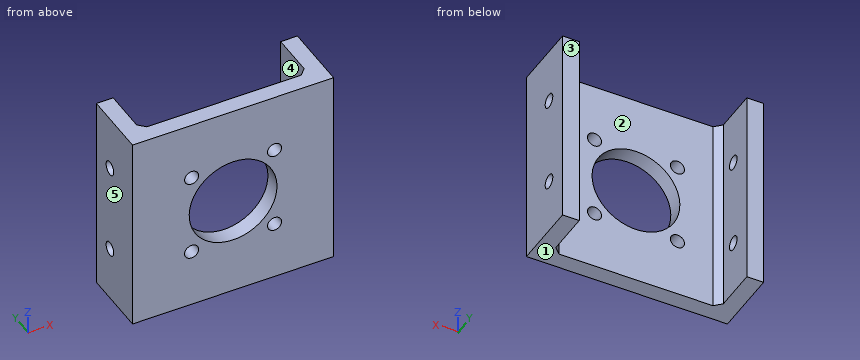
```python
from build123d import *

# Parameters (mm, degrees)
SKETCH_1_W           = 60
SKETCH_1_H           = 60
SKETCH_1_R           = 13.1
SKETCH_1_R_2         = 2.1
EXTRUDE_1_DEPTH      = 5
SKETCH_2_W           = 5
SKETCH_2_H           = 60
EXTRUDE_2_DEPTH      = 15
SKETCH_4_R           = 2.1
CUT_EXTRUDE_M4_DEPTH = 71
CHAMFER_1_SIZE       = 2


with BuildPart() as part:
    # 草图1 → 凸台-拉伸1 (new body)
    with BuildSketch(Plane(origin=(0, 0, 0), x_dir=(1, 0, 0), z_dir=(0, 1, 0))):
        Rectangle(SKETCH_1_W, SKETCH_1_H)
        with Locations(Location((0, 0, 0), (0, 0, 270))):
            Circle(SKETCH_1_R, mode=Mode.SUBTRACT)
        with Locations(Location((-12.374368671, -12.374368671, 0), (0, 0, 270))):
            Circle(SKETCH_1_R_2, mode=Mode.SUBTRACT)
        with Locations(Location((12.374368671, -12.374368671, 0), (0, 0, 90))):
            Circle(SKETCH_1_R_2, mode=Mode.SUBTRACT)
        with Locations(Location((-12.374368671, 12.374368671, 0), (0, 0, 90))):
            Circle(SKETCH_1_R_2, mode=Mode.SUBTRACT)
        with Locations(Location((12.374368671, 12.374368671, 0), (0, 0, 270))):
            Circle(SKETCH_1_R_2, mode=Mode.SUBTRACT)
    extrude(amount=EXTRUDE_1_DEPTH)

    # 草图2 → 凸台-拉伸2 (add)
    with BuildSketch(Plane(origin=(0, 5, 0), x_dir=(1, 0, 0), z_dir=(0, 1, 0))):
        with Locations((-27.5, 0)):
            Rectangle(SKETCH_2_W, SKETCH_2_H)
        with Locations((27.5, 0)):
            Rectangle(SKETCH_2_W, SKETCH_2_H)
    extrude(amount=EXTRUDE_2_DEPTH)

    # 草图4 → M4通孔 (cut, through all)
    with BuildSketch(Plane.ZY.offset(30)):
        with Locations((-13.5, 12.5)):
            Circle(SKETCH_4_R)
        with Locations(Location((13.5, 12.5, 0), (0, 0, 180))):
            Circle(SKETCH_4_R)
    extrude(amount=-CUT_EXTRUDE_M4_DEPTH, mode=Mode.SUBTRACT)

    # 倒角1
    chamfer_1_edges = [part.edges().sort_by_distance(p)[0] for p in [
        (-25, 5, 0),
        (25, 5, 0),
    ]]
    chamfer(chamfer_1_edges, length=CHAMFER_1_SIZE)


solid = part.part
```
Work out the finished part from the listing and answer in its coordinate system (mm). Face numbers are marked on the shaded views. A direction names the side the tool comes from. Round coordinates to 2 decimals unless told otherwise and drop trailing zeros. Write each loop counter-clockwise with the first axis right and the second up, starting at its lowest first coordinate (ties: lowest second). Pieces come first, ordered by that corner, then holes. Notation, with made-up numbers: (37.25, 83) - (64.25, 83) arc R21 cw to (64.25, 121) - close; hole circle Ø8 at (44.5, 58.5). An arc over 180 degrees is marked (long way). Return JSON: item names as keys, results as strings. Group by question number.
Q1. For the marked faces 1 and 2, determine the directions among +Z, -Z, +X, -X, +Y, -Y from which every point of the face is accessible in a straight line to the end or side of a thin tool.
Q2. The mould has two halves that part along X. Classify the marked faces 3, 4 and 5: released by +X, released by -X, zero draft, split by the parting line, or undercut.
Q3. Find the intervals of material crossed by L1, parallel to Y at x = 28.15, z = 13.5; L2, parallel to X at y = 4.75, z = 14; L3, parallel to X at y = 7.5, z = -19, in increasing order.
Q4. Each of these flat-tipped pins is pushed along its axis until it touches: pin 1 Ø2.5 at (x, z) = (12.37, -12.37) entering from +Y; pin 2 Ø5 at (x, z) = (3.5, 18.5) entering from +Y. Where does it stop, or does it pass through?
Q5. The part is cut by section B-B on z = 0. Write down the section's boundary in (x, y), then the cut area to 3 significant figures.
Q6. The part is cut by section A-A on y = 9.5. Write down the section's boundary in (x, z), then the cut area to 3 significant figures.
Q7. The part is cut by section D-D on x = -11.5. Write down the section's boundary in (y, z).
Q8. The part is cut by section C-C on x = 0. Write down the section's boundary in (y, z).
Solved:
{
 "1": {"face 1": "-Z, +X, -X, +Y, -Y", "face 2": "+Z, -Z, +Y"},
 "2": {"face 3": "zero draft", "face 4": "undercut", "face 5": "released by -X"},
 "3": {"L1": "0 to 10.4, 14.6 to 20", "L2": "-30 to -13.7, -11.04 to 11.04, 13.7 to 30", "L3": "-30 to -25, 25 to 30"},
 "4": {"pin 1": "through", "pin 2": "y = 5"},
 "5": {"outline": "(-30, 0) - (-13.1, 0) - (-13.1, 5) - (-23, 5) - (-25, 7) - (-25, 20) - (-30, 20) - close; (13.1, 0) - (30, 0) - (30, 20) - (25, 20) - (25, 7) - (23, 5) - (13.1, 5) - close", "area": "323 mm²"},
 "6": {"outline": "(-30, -30) - (-25, -30) - (-25, 30) - (-30, 30) - close; (25, -30) - (30, -30) - (30, 30) - (25, 30) - close", "area": "600 mm²"},
 "7": {"outline": "(0, -30) - (5, -30) - (5, -14.28) - (0, -14.28) - close; (0, -10.47) - (5, -10.47) - (5, -6.27) - (0, -6.27) - close; (0, 6.27) - (5, 6.27) - (5, 10.47) - (0, 10.47) - close; (0, 14.28) - (5, 14.28) - (5, 30) - (0, 30) - close"},
 "8": {"outline": "(0, -30) - (5, -30) - (5, -13.1) - (0, -13.1) - close; (0, 13.1) - (5, 13.1) - (5, 30) - (0, 30) - close"}
}
